from build123d import *

# Parameters (mm, degrees)
F0_W     = 74.3527244776
F0_H     = 107.3727235198
F0_R     = 8.4778544631
F0_R_2   = 7.9454205322
F1_DEPTH = 50.8
F3_DEPTH = 25.4
F4_DEPTH = 76.2
F6_DEPTH = 25.4


with BuildPart() as f1:
    # F0 (on Top) → F1 (new body)
    with BuildSketch(Plane.XY):
        with Locations((-6.234546192, 0.2309083939)):
            Rectangle(F0_W, F0_H)
        with Locations((-6.4654541202, -36.1372716725)):
            Circle(F0_R, mode=Mode.SUBTRACT)
        with Locations((-6.6963643767, 40.9863628447)):
            Circle(F0_R_2, mode=Mode.SUBTRACT)
    extrude(amount=F1_DEPTH)

    # F2 (on face) → F3 (join)
    with BuildSketch(Plane(origin=(-43.4109084308, 0, 0), x_dir=(0, -1, 0), z_dir=(-1, 0, 0))):
        with BuildLine():
            ThreePointArc((-27.3364075131, 50.8), (0, 23.4635924869), (27.3364075131, 50.8))
            Line((27.3364075131, 50.8), (15.4696153843, 50.8))
            ThreePointArc((15.4696153843, 50.8), (0, 35.3303846157), (-15.4696153843, 50.8))
            Line((-15.4696153843, 50.8), (-27.3364075131, 50.8))
        make_face()
    extrude(amount=F3_DEPTH)

    # F4 (cut): a face of the model
    f4_faces = [f1.faces().sort_by_distance(p)[0] for p in [
        (-43.4109084308, 0, 44.234491317),
    ]]
    extrude(f4_faces, amount=-F4_DEPTH, mode=Mode.SUBTRACT)

    # F5 (on face) → F6 (join)
    with BuildSketch(Plane.YZ.offset(30.9418160468)):
        with BuildLine():
            ThreePointArc((-25.9977905066, 50.8), (0, 24.8022094934), (25.9977905066, 50.8))
            Line((25.9977905066, 50.8), (15.4696153843, 50.8))
            ThreePointArc((15.4696153843, 50.8), (0, 35.3303846157), (-15.4696153843, 50.8))
            Line((-15.4696153843, 50.8), (-25.9977905066, 50.8))
        make_face()
    extrude(amount=F6_DEPTH)


solid = f1.part
Can you work these out from the model? Positions are in its coordinate system, mm. A direction names the side the tool comes from. Coordinates: 2 decimals unless noted, no trailing zeros. Write each loop counter-clockwise with the first axis right and the second up, starting at its lowest first coordinate (ties: lowest second). Pieces come first, ordered by that corner, then holes. Notation, with made-up numbers: (80.25, 55.25) -> (115.25, 55.25) arc R20 cw to (115.25, 85.25) -> close; hole circle Ø10 at (80, 33.5). An arc over 180 degrees is marked (long way). Write item = value, one per line.
(1) Thinking about a two-plate mould opening in Y: for faces 1 (the face through (-55.93, 0.6, 23.47)), 2 (the face through (-7.111, 0.34, 35.334)), 3 (the face through (-7, 53.917, 25)), which applies, +Y half, -Y half, draft (parallel to the pull), parting line (faces both ways), or undercut?
Verdict:
face_1 = parting line
face_2 = undercut
face_3 = +Y half
(2) Imagine slicing it at B-B (x = -10.5). Please give me the cut outline in (y, z), and give its area (3 significant figures).
Verdict:
outline = (-53.46, 0) -> (-43.59, 0) -> (-43.59, 50.8) -> (-53.46, 50.8) -> close; (-28.68, 0) -> (34.01, 0) -> (34.01, 50.8) -> (15.47, 50.8) arc R15.47 cw to (-15.47, 50.8) -> (-28.68, 50.8) -> close; (47.96, 0) -> (53.92, 0) -> (53.92, 50.8) -> (47.96, 50.8) -> close
area = 3,610 mm^2
(3) Imagine slicing it at A-A (y = 43). Please give me the cut outline in (x, z).
Verdict:
outline = (-43.41, 0) -> (-14.38, 0) -> (-14.38, 50.8) -> (-43.41, 50.8) -> close; (0.99, 0) -> (30.94, 0) -> (30.94, 50.8) -> (0.99, 50.8) -> close
(4) On a 3-axis mill with a long thin cutter (end or side, diameter ignored), from which of +Z, -Z, +X, -X, +Y, -Y can I reach the whole of each face in a straight line? I mean faces 4 (the face through (30.942, -1, 19)), 5 (the face through (-43.411, -1, 19)), 6 (the face through (-7, 1, 0)). Say none if no direction works.
Verdict:
face_4 = -Z, +X
face_5 = -Z, -X
face_6 = -Z, +X, -X, +Y, -Y
(5) If I drill on probe 1 along X at (y, z) = (-36.5, 41.5); probe 2 along X at (y, z) = (28, 10.5); probe 3 along X at (y, z) = (40, 6.5), over which ranges is the centre line in solid material (lowest first)?
Verdict:
probe_1 = -43.41 to -14.94, 2 to 30.94
probe_2 = -43.41 to 30.94
probe_3 = -43.41 to -14.58, 1.19 to 30.94
(6) Imagine slicing it at C-C (z = 46). Please give me the cut outline in (x, y), and give its area (3 significant figures).
Verdict:
outline = (-68.81, -26.91) -> (-43.41, -26.91) -> (-43.41, -53.46) -> (30.94, -53.46) -> (30.94, -25.55) -> (56.34, -25.55) -> (56.34, -14.71) -> (-68.81, -14.71) -> close; (-68.81, 14.71) -> (56.34, 14.71) -> (56.34, 25.55) -> (30.94, 25.55) -> (30.94, 53.92) -> (-43.41, 53.92) -> (-43.41, 26.91) -> (-68.81, 26.91) -> close; hole circle Ø16.96 at (-6.47, -36.14); hole circle Ø15.89 at (-6.7, 40.99)
area = 6,540 mm^2
(7) For pin 1 (15.5 mm diameter, centred on x = -6.47, y = -36.14, fed in from -Z); pin 2 (1 mm diameter, centred on y = -39.5, z = 41, fed in from -X); pin 3 (6 mm diameter, centred on x = -43, y = 7, fed in from -Z), each with a flat end and sliding along its axis, tell me the tip position at first contact or that it passes through.
Verdict:
pin_1 = through
pin_2 = -43.41
pin_3 = 0
(8) Imagine slicing it at D-D (y = 0). Please give me the cut outline in (x, z), and give its area (3 significant figures).
Verdict:
outline = (-68.81, 23.46) -> (-43.41, 23.46) -> (-43.41, 0) -> (30.94, 0) -> (30.94, 24.8) -> (56.34, 24.8) -> (56.34, 35.33) -> (-68.81, 35.33) -> close
area = 3,200 mm^2
